from build123d import *

# Parameters (mm, degrees)
SKETCH1_W                                       = 35
SKETCH1_H                                       = 8
BOSS_EXTRUDE1_DEPTH                             = 6
SKETCH2_W                                       = 4.6
SKETCH2_H                                       = 3
CUT_EXTRUDE1_DEPTH                              = 5
CSK_FOR_M3_FLAT_HEAD_MACHINE_SCREW1_D           = 3.2
CSK_FOR_M3_FLAT_HEAD_MACHINE_SCREW1_CSINK_D     = 6.3
CSK_FOR_M3_FLAT_HEAD_MACHINE_SCREW1_CSINK_ANGLE = 90


with BuildPart() as part:
    # Sketch1 → Boss-Extrude1 (new body)
    with BuildSketch(Plane(origin=(0, 0, 0), x_dir=(1, 0, 0), z_dir=(0, 1, 0))):
        Rectangle(SKETCH1_W, SKETCH1_H)
    extrude(amount=-BOSS_EXTRUDE1_DEPTH)

    # Sketch2 → Cut-Extrude1 (cut)
    with BuildSketch(Plane.XY.offset(4)):
        with Locations((0, -3)):
            Rectangle(SKETCH2_W, SKETCH2_H)
    extrude(amount=-CUT_EXTRUDE1_DEPTH, mode=Mode.SUBTRACT)

    # CSK for M3 Flat Head Machine Screw1 (through all)
    with Locations(Plane(origin=(-14, 0, 0), x_dir=(0, 0, 1), z_dir=(0, 1, 0))):
        with Locations((0, 0), (0, 28)):
            CounterSinkHole(CSK_FOR_M3_FLAT_HEAD_MACHINE_SCREW1_D / 2, CSK_FOR_M3_FLAT_HEAD_MACHINE_SCREW1_CSINK_D / 2, counter_sink_angle=CSK_FOR_M3_FLAT_HEAD_MACHINE_SCREW1_CSINK_ANGLE)


solid = part.part
The listing builds one solid part. Answer for the finished solid, in the listing's coordinates (mm). A direction names the side the tool comes from. Coordinates: 2 decimals unless noted, no trailing zeros. Order: outer loops, then holes, each group sorted by start corner. A loop starts at its lowest first (then second) coordinate and runs counter-clockwise, first axis right, second up. Notation, with made-up numbers: M -14,55 L 14,55 A18 ccw 14,64 Z; hole C 69.25,14 d7. An arc over 180 degrees is marked long. Use CSV: the item, a comma, the result in double quotes.
Q1. Given pin 1 Ø1 at (x, y) = (-2, -3) entering from +Z, flat-ended and moving along its own axis, determine where the tip first touches the part or whether it passes through.
Here are the results:
pin 1,"z = 4"
Q2. Determine the mould class of faces 1 (the flat face through (0, -1, 4)), 2 (the cylindrical face through (15.586, -3.806, 0.208)), 3 (the flat face through (17.5, -3, 0)) for opening direction Z: pulls with the +Z half, pulls with the -Z half, needs draft (parallel to the pull), parting line crosses it, or undercut.
Here are the results:
face 1,"pulls with the +Z half"
face 2,"undercut"
face 3,"needs draft"
Q3. Straight lines are drawn through the part: L1, parallel to X at y = -3.9, z = 0; L2, parallel to X at y = -4.7, z = 0; L3, parallel to X at y = -0.9, z = 1.5. For each, find the intervals that lie inside material, in ascending order.
Here are the results:
L1,"-17.5 to -15.6, -12.4 to -2.3, 2.3 to 12.4, 15.6 to 17.5"
L2,"-17.5 to -15.6, -12.4 to 12.4, 15.6 to 17.5"
L3,"-17.5 to -15.68, -12.32 to 12.32, 15.68 to 17.5"
Q4. A tool of negligible diameter and unlimited length cuts with its end or side. For faces 4 (the flat face through (0, -1.5, 2)), 5 (the flat face through (0, -6, 0)), from which of +Z, -Z, +X, -X, +Y, -Y can it reach the whole face along a straight path? Write none if from no direction.
Here are the results:
face 4,"+Z"
face 5,"+Z, -Z, +X, -X, -Y"
Q5. Section C-C (y = -0.65) is taken. Determine the outline of the cut face in (x, z).
Here are the results:
outline,"M -17.5,-4 L 17.5,-4 L 17.5,4 L -17.5,4 Z; hole C -14,0 d5; hole C 14,0 d5"
Q6. Section A-A (z = 0) is taken. Determine the outline of the cut face in (x, y).
Here are the results:
outline,"M -17.5,-6 L -15.6,-6 L -15.6,-1.55 L -17.15,0 L -17.5,0 Z; M -12.4,-6 L 12.4,-6 L 12.4,-1.55 L 10.85,0 L -10.85,0 L -12.4,-1.55 Z; M 15.6,-6 L 17.5,-6 L 17.5,0 L 17.15,0 L 15.6,-1.55 Z; hole M -2.3,-4.5 L 2.3,-4.5 L 2.3,-1.5 L -2.3,-1.5 Z"
Q7. Section B-B (x = 14) is taken. Determine the outline of the cut face in (y, z), then the cut area to 3 significant figures.
Here are the results:
outline,"M -6,-4 L 0,-4 L 0,-3.15 L -1.55,-1.6 L -6,-1.6 Z; M -6,1.6 L -1.55,1.6 L 0,3.15 L 0,4 L -6,4 Z"
area,"26.4 mm2"
